Verification items for the finished model (mm, model axes). A direction names the side the tool comes from. Give positions to 0.01 mm unless a question says otherwise; leave off trailing zeros. Write each loop counter-clockwise with the first axis right and the second up, starting at its lowest first coordinate (ties: lowest second). Pieces come first, ordered by that corner, then holes. Notation, with made-up numbers: (78.25, 18.25) -> (85.25, 18.25) arc R22 cw to (85.25, 50.25) -> close; hole circle Ø10 at (49, 75). An arc over 180 degrees is marked (long way). Answer as CSV lines item,"result". Start each with the question number.
1) Sectioned sample at C-C on z = 7.25. Record the cut outline in (x, y), and give its area (3 significant figures).
2) Sectioned sample at D-D on x = 10.5. Record the cut outline in (y, z).
3) Sectioned sample at B-B on y = 22. Record the cut outline in (x, z), and give its area (3 significant figures).
4) Material ranges on L1, parallel to Y at x = 15, z = 6.5; L2, parallel to Y at x = -1, z = 3; L3, parallel to Z at x = -41, y = -8, recorded low to high.
5) Sectioned sample at A-A on x = -5. Record the cut outline in (y, z), and give its area (3 significant figures).
6) Tool access check on faces 4 (the flat face through (-17, -9.648, 4)), 5 (the flat face through (10, 10, 16.199)), 6 (the flat face through (10, -12.148, 4)), 7 (the flat face through (10, 10, -8.801)), 8 (the flat face through (-25, 0.852, -10)). Record the directions out of +Z, -Z, +X, -X, +Y, -Y that give a thin tool (end or side, any length) a straight path to the whole face; none if there is none.
7) Mould release check, pull along Y, two halves, no side actions. Record for faces 1 (the flat face through (-38, 1.013, -10)), 2 (the flat face through (10, 32.852, 4)), 3 (the flat face through (-25, 10, -11.301)): released by +Y, released by -Y, zero draft, split by the parting line, or undercut.
8) Gauge pin test, flat ends, axial feed: pin 1 Ø2 at (x, z) = (-25.5, -10) entering from -Y; pin 2 Ø2 at (x, z) = (-38, -10.5) entering from +Y; pin 3 Ø1.6 at (x, z) = (-25, -10) entering from +Y. Record the tip position at first contact, or that the pin passes through.
```python
from build123d import *

# Parameters (mm, degrees)
F0_W        = 49.9999988824
F0_H        = 29.9999988824
F0_W_2      = 45.0000008941
F0_H_2      = 25.0000008941
F0_W_3      = 40
F0_H_3      = 20
F1_DEPTH    = 60
F2_DEPTH    = 55
F3_DEPTH    = 25
F4_T1_DEPTH = 50.7168307737
F4_T3_DEPTH = 70.7168307737
F5_R        = 3
F7_DEPTH    = 2


# Not quite as in the source:
# - a fillet or chamfer that OpenCascade refuses, or shapes differently, is made with other operations: its cross-section is extruded or revolved along the edge and cut away or added


with BuildPart() as f1:
    # F0 (on Right) → F1 (new body)
    with BuildSketch(Plane.YZ):
        with Locations((10.3521584719, 3.6993094161)):
            Rectangle(F0_W, F0_H)
        with Locations((10.3521584719, 3.6993094161)):
            Rectangle(F0_W_2, F0_H_2, mode=Mode.SUBTRACT)
        with Locations((10.3521584719, 3.6993094161)):
            Rectangle(F0_W_2, F0_H_2)
        with Locations((10.3521584719, 3.6993094161)):
            Rectangle(F0_W_3, F0_H_3, mode=Mode.SUBTRACT)
        with Locations((10.3521584719, 3.6993094161)):
            Rectangle(F0_W_3, F0_H_3)
    extrude(amount=-F1_DEPTH)

    # F0 (on Right) → F2 (cut)
    with BuildSketch(Plane.YZ):
        with Locations((10.3521584719, 3.6993094161)):
            Rectangle(F0_W_3, F0_H_3)
    extrude(amount=-F2_DEPTH, mode=Mode.SUBTRACT)

    # F0 (on Right) → F3 (join)
    with BuildSketch(Plane.YZ):
        with Locations((10.3521584719, 3.6993094161)):
            Rectangle(F0_W_2, F0_H_2)
        with Locations((10.3521584719, 3.6993094161)):
            Rectangle(F0_W_3, F0_H_3, mode=Mode.SUBTRACT)
    extrude(amount=F3_DEPTH)

    # F4: chamfer of 5 on 4 edges, made by hand

    # F4_s2 → F4_t1 (cut)
    with BuildSketch(Plane.XY.offset(-21.6591059707)):
        Polygon((25, -7.1478419751), (20, -12.1478419751), (25, -12.1478419751), align=None)
        Polygon((25, 27.852158919), (20, 32.852158919), (25, 32.852158919), align=None)
    extrude(amount=F4_T1_DEPTH, mode=Mode.SUBTRACT)

    # F4_s4 → F4_t3 (cut)
    with BuildSketch(Plane.XZ.offset(-45.7105738588)):
        Polygon((20, -8.8006910309), (25, -3.8006910309), (25, -8.8006910309), align=None)
        Polygon((25, 11.1993098632), (20, 16.1993098632), (25, 16.1993098632), align=None)
    extrude(amount=F4_T3_DEPTH, mode=Mode.SUBTRACT)

    # F5
    f5_edges = [f1.edges().sort_by_distance(p)[0] for p in [
        (-30, 35.352158, -11.30069),
        (-30, 35.352158, 18.699309),
        (-30, -14.647841, -11.30069),
        (-30, -14.647841, 18.699309),
    ]]
    fillet(f5_edges, radius=F5_R)

    # F6 (on face) → F7 (cut)
    with BuildSketch(Plane(origin=(0, 0, -11.3006900251), x_dir=(1, 0, 0), z_dir=(0, 0, -1))):
        with BuildLine():
            Line((-40.5811635508, -19.8521577269), (-36.5980909465, -19.8521577269))
            Line((-36.5980909465, -19.8521577269), (-36.5980909465, -1.0129664961))
            Line((-36.5980909465, -1.0129664961), (-39.8719622175, -1.0129664961))
            Line((-39.8719622175, -1.0129664961), (-45.941406186, -5.8454313948))
            Line((-45.941406186, -5.8454313948), (-44.0199653644, -8.2410475264))
            Line((-44.0199653644, -8.2410475264), (-41.8552519925, -6.5010303018))
            add(Edge.make_bspline(
                [(-40.4780819617, -5.2022022786), (-41.4676652174, -6.1917855343), (-41.8552519925, -6.5010303018)],
                knots=[0, 0, 0, 1, 1, 1], degree=2))
            Line((-40.4780819617, -5.2022022786), (-40.5399309151, -7.1607524722))
            Line((-40.5399309151, -7.1607524722), (-40.5811635508, -8.9502488597))
            Line((-40.5811635508, -8.9502488597), (-40.5811635508, -19.8521577269))
        make_face()
        with BuildLine():
            Line((-26.8667704258, -19.8521577269), (-22.8777154217, -19.8521577269))
            add(Edge.make_bspline(
                [(-19.9318596147, -17.7389851496), (-21.0133994036, -19.326806957), (-22.8777154217, -19.8521577269)],
                knots=[0, 0, 0, 0.6691374514, 0.6691374514, 0.6691374514], degree=2))
            add(Edge.make_bspline(
                [(-18.315540297, -10.4346237433), (-18.315540297, -15.3660469676), (-19.9318596147, -17.7389851496)],
                knots=[0, 0, 0, 1, 1, 1], degree=2))
            add(Edge.make_bspline(
                [(-19.9834004093, -3.1900496586), (-18.315540297, -5.664007798), (-18.315540297, -10.4346237433)],
                knots=[0, 0, 0, 1, 1, 1], degree=2))
            add(Edge.make_bspline(
                [(-23.4706324827, -0.852159217), (-21.2601126538, -1.2962861316), (-19.9834004093, -3.1900496586)],
                knots=[0.234520788, 0.234520788, 0.234520788, 1, 1, 1], degree=2))
            Line((-23.4706324827, -0.852159217), (-26.4191418917, -0.852159217))
            add(Edge.make_bspline(
                [(-29.8730480712, -3.0807831742), (-28.6475822393, -1.2833288146), (-26.4191418917, -0.852159217)],
                knots=[0, 0, 0, 0.7601220886, 0.7601220886, 0.7601220886], degree=2))
            add(Edge.make_bspline(
                [(-31.4852441253, -10.4346237433), (-31.4852441253, -5.445474829), (-29.8730480712, -3.0807831742)],
                knots=[0, 0, 0, 1, 1, 1], degree=2))
            add(Edge.make_bspline(
                [(-29.8297538037, -17.6627047736), (-31.4852441253, -15.2134862157), (-31.4852441253, -10.4346237433)],
                knots=[0, 0, 0, 1, 1, 1], degree=2))
            add(Edge.make_bspline(
                [(-26.8667704258, -19.8521577269), (-28.7134061438, -19.3142876129), (-29.8297538037, -17.6627047736)],
                knots=[0.3256694736, 0.3256694736, 0.3256694736, 1, 1, 1], degree=2))
        make_face()
        with BuildLine():
            add(Edge.make_bspline(
                [(-27.5269111024, -10.4346237433), (-27.5269111024, -13.8981651383), (-26.9290378854, -15.3990330761)],
                knots=[0, 0, 0, 1, 1, 1], degree=2))
            add(Edge.make_bspline(
                [(-26.92285299, -5.4537213561), (-27.5269111024, -6.9669590847), (-27.5269111024, -10.4346237433)],
                knots=[0, 0, 0, 1, 1, 1], degree=2))
            add(Edge.make_bspline(
                [(-24.9127620019, -3.9404836276), (-26.3187948777, -3.9404836276), (-26.92285299, -5.4537213561)],
                knots=[0, 0, 0, 1, 1, 1], degree=2))
            add(Edge.make_bspline(
                [(-22.908855909, -5.4537213561), (-23.535591971, -3.9404836276), (-24.9127620019, -3.9404836276)],
                knots=[0, 0, 0, 1, 1, 1], degree=2))
            add(Edge.make_bspline(
                [(-22.2821198471, -10.4346237433), (-22.2821198471, -6.9669590847), (-22.908855909, -5.4537213561)],
                knots=[0, 0, 0, 1, 1, 1], degree=2))
            add(Edge.make_bspline(
                [(-22.9006093819, -15.3804783901), (-22.2821198471, -13.8610557662), (-22.2821198471, -10.4346237433)],
                knots=[0, 0, 0, 1, 1, 1], degree=2))
            add(Edge.make_bspline(
                [(-24.9127620019, -16.899901014), (-23.5190989167, -16.899901014), (-22.9006093819, -15.3804783901)],
                knots=[0, 0, 0, 1, 1, 1], degree=2))
            add(Edge.make_bspline(
                [(-26.9290378854, -15.3990330761), (-26.3311646684, -16.899901014), (-24.9127620019, -16.899901014)],
                knots=[0, 0, 0, 1, 1, 1], degree=2))
        make_face(mode=Mode.SUBTRACT)
    extrude(amount=-F7_DEPTH, mode=Mode.SUBTRACT)


solid = f1.part
```
Ans:
1,outline,"(-60, -14.65) -> (0, -14.65) -> (0, -12.15) -> (20, -12.15) -> (22.5, -9.65) -> (-55, -9.65) -> (-55, 30.35) -> (22.5, 30.35) -> (20, 32.85) -> (0, 32.85) -> (0, 35.35) -> (-60, 35.35) -> close"
1,area,"906 mm²"
2,outline,"(-12.15, -8.8) -> (32.85, -8.8) -> (32.85, 16.2) -> (-12.15, 16.2) -> close; hole (-9.65, -6.3) -> (30.35, -6.3) -> (30.35, 13.7) -> (-9.65, 13.7) -> close"
3,outline,"(-60, -11.3) -> (0, -11.3) -> (0, -8.8) -> (20, -8.8) -> (22.5, -6.3) -> (-55, -6.3) -> (-55, 13.7) -> (22.5, 13.7) -> (20, 16.2) -> (0, 16.2) -> (0, 18.7) -> (-60, 18.7) -> close"
3,area,"806 mm²"
4,L1,"y = -12.15 to -9.65, 30.35 to 32.85"
4,L2,"y = -14.65 to -9.65, 30.35 to 35.35"
4,L3,"z = -11.3 to -6.3, 13.7 to 18.7"
5,outline,"(-14.65, -8.3) arc R3 ccw to (-11.65, -11.3) -> (32.35, -11.3) arc R3 ccw to (35.35, -8.3) -> (35.35, 15.7) arc R3 ccw to (32.35, 18.7) -> (-11.65, 18.7) arc R3 ccw to (-14.65, 15.7) -> close; hole (-9.65, -6.3) -> (30.35, -6.3) -> (30.35, 13.7) -> (-9.65, 13.7) -> close"
5,area,"692 mm²"
6,face 4,"+X"
6,face 5,"+Z, +X, +Y, -Y"
6,face 6,"+Z, -Z, +X, -Y"
6,face 7,"-Z, +X, +Y, -Y"
6,face 8,"-Z"
7,face 1,"undercut"
7,face 2,"released by +Y"
7,face 3,"zero draft"
8,pin 1,"stops at y = -14.57"
8,pin 2,"stops at y = 35.1"
8,pin 3,"stops at y = 35.21"
